Autodesk Inventor part; units mm, degrees
ref_plane "YZ Plane" through (0, 0, 0) normal (1, 0, 0) x (0, 1, 0)
ref_plane "XZ Plane" through (0, 0, 0) normal (0, 1, 0) x (-1, 0, 0)
ref_plane "XY Plane" through (0, 0, 0) normal (0, 0, 1) x (1, 0, 0)
sketch "Sketch1" plane through (0, 0, 0) normal (1, 0, 0) x (0, 1, 0)
  line L0 (48, 50) -> (-48, 50)
  line L1 (-48, 50) -> (-48, -50)
  line L2 (-48, -50) -> (48, -50)
  line L3 (48, -50) -> (48, 50)
  point P0 (0, 0)
  dimension "d0" = 96
  dimension "d1" = 100
  dimension "d2" = 50
  dimension "d3" = 48
extrude "Extrusion1" add sketch "Sketch1" along normal blind 1.5
sketch "Sketch2" plane through (0, -48, 50) normal (0, 0, 1) x (1, 0, 0)
  line L0 (0, 96) -> (1.5, 96)
  line L1 (1.5, 96) -> (-7, 96)
  line L2 (-7, 96) -> (-7, 0)
  line L3 (-7, 0) -> (1.5, 0)
  line L4 (1.5, 0) -> (1.5, 96)
  point P0 (0, 48)
  dimension "d6" = 8.5
  dimension "d7" = 96
extrude "Extrusion2" add sketch "Sketch2" against normal blind 1.5
mirror "Mirror1" about plane through (0, 0, 0) normal (0, 0, 1) of "Extrusion2"
fillet "Fillet1" radius 0.5 2 edges at (1.5, 0, 50) (1.5, 0, -50)
sketch "Sketch12" plane through (-7, -48, 48.5) normal (0, -1, 0) x (1, 0, 0)
  arc A0 (8, -98.5) -> (8.5, -98) centre (8, -98) ccw
  line L0 (8.5, 1) -> (8.5, -98)
  arc A1 (8.5, 1) -> (8, 1.5) centre (8, 1) ccw
  line L1 (0, 1.5) -> (8, 1.5)
  line L2 (0, 1.5) -> (0, 0)
  line L3 (7, 0) -> (0, 0)
  line L4 (7, 0) -> (7, -97)
  line L5 (7, -97) -> (0, -97)
  line L6 (0, -98.5) -> (0, -97)
  line L7 (0, -98.5) -> (8, -98.5)
  point P0 (7, -48.5)
extrude "Extrusion8" add sketch "Sketch12" along normal blind 56.75
sketch "Sketch13" plane through (-7, 48, 48.5) normal (0, 1, 0) x (1, 0, 0)
  arc A0 (8.5, 98) -> (8, 98.5) centre (8, 98) ccw
  line L0 (0, 98.5) -> (8, 98.5)
  line L1 (0, 98.5) -> (0, 97)
  line L2 (0, 97) -> (7, 97)
  line L3 (7, 97) -> (7, 0)
  line L4 (0, 0) -> (7, 0)
  line L5 (0, -1.5) -> (0, 0)
  line L6 (8, -1.5) -> (0, -1.5)
  arc A1 (8, -1.5) -> (8.5, -1) centre (8, -1) ccw
  line L7 (8.5, 98) -> (8.5, -1)
  point P0 (7, 48.5)
extrude "Extrusion9" add sketch "Sketch13" along normal blind 56.75
sketch "Sketch14" plane through (1.5, 0, 0) normal (1, 0, 0) x (0, 0, -1)
  line L0 (49.5, -104.75) -> (49.5, 104.75)
  line L1 (-49.5, 104.75) -> (49.5, 104.75)
  line L2 (-49.5, 104.75) -> (-49.5, -104.75)
  line L3 (49.5, -104.75) -> (-49.5, -104.75)
  line L4 (0, 0) -> (-23.5475, 0) construction
  point P0 (35, -100.75)
  point P1 (-35, -100.75)
  point P2 (35, 100.75)
  point P3 (-35, 100.75)
  dimension "d88" = 70
  dimension "d89" = 35
  dimension "d90" = 4
hole "Hole6" at (1.5, -100.75, -35) at (1.5, -100.75, 35) at (1.5, 100.75, -35) at (1.5, 100.75, 35) direction (-1, 0, 0) diameter 3.454 end through all
sketch "Sketch15" plane through (1.5, 0, 0) normal (1, 0, 0) x (0, 0, -1)
  circle A0 centre (-35, 100.75) radius 1.727
  line L0 (0, 0) -> (0, 19.4005) construction
  line L1 (0, 0) -> (22.6917, 0) construction
  point P0 (-27.5, 51.25)
  point P1 (-27.5, -51.25)
  point P2 (27.5, 51.25)
  point P3 (27.5, -51.25)
  dimension "d150" = 7.5
  dimension "d167" = 102.5
  dimension "d168" = 51.25
hole "Hole7" at (1.5, 51.25, 27.5) at (1.5, -51.25, 27.5) at (1.5, -51.25, -27.5) at (1.5, 51.25, -27.5) direction (-1, 0, 0) diameter 3.454 end through all
sketch "Sketch16" plane through (0, 0, 0) normal (-1, 0, 0) x (0, 0, 1)
  line L0 (36.5, 68.75) -> (48.5, 68.75)
  line L1 (48.5, 68.75) -> (48.5, 84.75)
  line L2 (48.5, 84.75) -> (36.5, 84.75)
  line L3 (36.5, 84.75) -> (36.5, 68.75)
  circle A0 centre (-35, 100.75) radius 1.727
  circle A1 centre (-35, -100.75) radius 1.727
  circle A2 centre (35, -100.75) radius 1.727
  circle A3 centre (35, 100.75) radius 1.727
  line L4 (-48.5, 104.75) -> (-48.5, -104.75)
  line L5 (48.5, -104.75) -> (-48.5, -104.75)
  line L6 (48.5, -104.75) -> (48.5, 104.75)
  line L7 (-48.5, 104.75) -> (48.5, 104.75)
  line L8 (48.5, -104.75) -> (48.5, 104.75)
  circle A4 centre (27.5, 51.25) radius 1.727
  point P0 (0, 0)
  dimension "d105" = 12
  dimension "d106" = 16
  dimension "d170" = 20
extrude "Extrusion10" add sketch "Sketch16" along normal blind 0.8 contours L3 L2 L1 L0
sketch "Sketch17" plane through (-0.8, 0, 0) normal (-1, 0, 0) x (0, 0, 1)
  line L0 (36.5, 68.75) -> (48.5, 68.75)
  line L1 (48.5, 84.75) -> (48.5, 68.75)
  line L2 (48.5, 84.75) -> (36.5, 84.75)
  line L3 (36.5, 84.75) -> (36.5, 68.75)
  line L4 (36.5, 68.75) -> (48.5, 68.75)
  line L5 (36.5, 68.75) -> (36.5, 84.75)
  point P0 (0, 0)
  point P1 (39.5, 72)
  point P2 (39.5, 81.5)
  point P3 (36.5, 76.75)
  dimension "d110" = 9.5
  dimension "d123" = 9
  dimension "d152" = 4.75
hole "Hole8" at (-0.8, 72, 39.5) at (-0.8, 81.5, 39.5) direction (1, 0, 0) diameter 2.2 end through all
chamfer "Chamfer2" distance 2 angle 45 2 edges at (-0.4, 68.75, 36.5) (-0.4, 84.75, 36.5)
sketch "Sketch22" plane through (1.5, 0, 0) normal (1, 0, 0) x (0, 0, -1)
  line L0 (41.5, -104.75) -> (50, -104.75)
  line L1 (50, -104.75) -> (50, 104.75)
  line L2 (50, 104.75) -> (41.5, 104.75)
  line L3 (41.5, 104.75) -> (41.5, -104.75)
  line L4 (50, -104.75) -> (50, 104.75)
  line L5 (-49.5, 104.75) -> (49.5, 104.75)
  point P0 (0, 0)
  point P1 (50, 0)
  point P2 (45.75, 104.75)
  dimension "d146" = 8.5
extrude "Extrusion13" cut sketch "Sketch22" against normal through all
sketch "Sketch24" plane through (0, -48, 48.5) normal (0, 0, -1) x (-1, 0, 0)
  line L0 (0, 132.75) -> (0.8, 132.75)
  line L1 (0.8, 132.75) -> (7, 132.75)
  line L2 (7, 132.75) -> (7, 116.75)
  line L3 (7, 116.75) -> (0.8, 116.75)
  line L4 (0.8, 116.75) -> (0.8, 132.75)
  line L5 (0.8, 116.75) -> (0, 116.75)
  line L6 (0, -56.75) -> (0, 116.75)
  line L7 (7, -56.75) -> (0, -56.75)
  line L8 (7, 152.75) -> (7, -56.75)
  line L9 (0, 152.75) -> (7, 152.75)
  line L10 (0, 132.75) -> (0, 152.75)
  line L11 (0, 132.75) -> (0.8, 132.75)
  line L12 (0.8, 132.75) -> (0.8, 116.75)
  line L13 (7, 152.75) -> (7, -56.75)
  point P0 (0, 48)
  point P1 (7, 124.75)
  dimension "d160" = 16
extrude "Extrusion15" cut sketch "Sketch24" against normal through all contours L1 L2 L3 L4
sketch "Sketch25" plane through (1.5, 0, 0) normal (1, 0, 0) x (0, 0, -1)
  line L0 (41.5, -104.75) -> (41.5, 104.75)
  line L1 (-49.5, 104.75) -> (41.5, 104.75)
  line L2 (-49.5, 104.75) -> (-49.5, -104.75)
  line L3 (41.5, -104.75) -> (-49.5, -104.75)
  circle A0 centre (-39.5, 72) radius 1.1
  circle A1 centre (-39.5, 81.5) radius 1.1
  circle A2 centre (27.5, -51.25) radius 1.727
  circle A3 centre (-27.5, 51.25) radius 1.727
  circle A4 centre (-27.5, -51.25) radius 1.727
  circle A5 centre (27.5, 51.25) radius 1.727
  circle A6 centre (35, 100.75) radius 1.727
  circle A7 centre (35, -100.75) radius 1.727
  circle A8 centre (-35, -100.75) radius 1.727
  circle A9 centre (-35, 100.75) radius 1.727
  line L4 (0, 0) -> (-27.5, 0) construction
  point P0 (38, 93.75)
  point P1 (-38, 93.75)
  point P2 (38, -93.75)
  point P3 (-38, -93.75)
  dimension "d171" = 76
  dimension "d172" = 38
  dimension "d180" = 7
hole "Hole10" at (1.5, 93.75, -38) at (1.5, 93.75, 38) at (1.5, -93.75, -38) at (1.5, -93.75, 38) direction (-1, 0, 0) diameter 3.454 end through all
properties part number "FR-Default" material "Aluminum 6061"
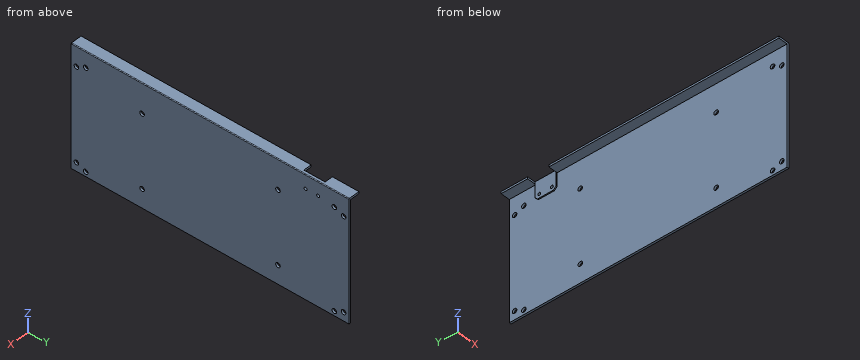
Input: part model. Units: mm. Frame: model coordinates. Round coordinates to 2 decimals unless told otherwise and drop trailing zeros. Loops run counter-clockwise (first coordinate to the right, second up) from the corner with the lowest first, then second, coordinate; pieces in that order, holes last. Notation, with made-up numbers: M 59.25,29.25 L 115.25,29.25 A25 ccw 115.25,68.25 Z; hole C 89.5,29.5 d6. An arc over 180 degrees is marked long. Answer as CSV lines item,"result". Start each with the question number.
(1) First-contact query: pin 1 (7 mm diameter, centred on y = 75.5, z = 43, fed in from -X); pin 2 (2 mm diameter, centred on x = -4, y = -77, fed in from -Z); pin 3 (10 mm diameter, centred on y = -36.5, z = -10, fed in from -X); pin 4 (5.5 mm diameter, centred on y = -93.75, z = 38, fed in from +X). Flat tips, straight axial feed; report the tip coordinate or a pass-through.
(2) Section C-C, the plane z = 2. Output: boundary loops of the cut face in (x, y), plus the area to 3 significant figures.
(3) Line query: line 1 (Z direction, x = 1.05, y = -51.25); line 2 (Y direction, x = 0.8, z = -38); line 3 (Z direction, x = 0.95, y = 81.5). Output: solid intervals per line, ascending. Write a range as [from, to].
(4) Section A-A, the plane x = -4.75. Output: boundary loops of the cut face in (y, z).
(5) Section B-B, the plane y = 1. Output: boundary loops of the cut face in (x, z).
Values found:
1,pin 1,"stops at x = -0.8"
1,pin 2,"stops at z = 48.5"
1,pin 3,"stops at x = 0"
1,pin 4,"stops at x = 1.5"
2,outline,"M 0,-104.75 L 1.5,-104.75 L 1.5,104.75 L 0,104.75 Z"
2,area,"314 mm²"
3,line 1,"z = [-41.5, -29.23], [-25.77, 25.77], [29.23, 50]"
3,line 2,"y = [-104.75, -95.48], [-92.02, 92.02], [95.48, 104.75]"
3,line 3,"z = [-41.5, 38.4], [40.6, 50]"
4,outline,"M -104.75,48.5 L 68.75,48.5 L 68.75,50 L -104.75,50 Z; M 84.75,48.5 L 104.75,48.5 L 104.75,50 L 84.75,50 Z"
5,outline,"M -7,48.5 L 0,48.5 L 0,-41.5 L 1.5,-41.5 L 1.5,49.5 A0.5 ccw 1,50 L -7,50 Z"
